Geometry: final body of the model. Coordinates: model frame, mm. Face numbers are marked on the shaded views. Round coordinates to 2 decimals unless told otherwise and drop trailing zeros. Order: outer loops, then holes, each group sorted by start corner. A loop starts at its lowest first (then second) coordinate and runs counter-clockwise, first axis right, second up. Notation, with made-up numbers: M 56.5,69 L 65.5,69 A21 cw 65.5,108 Z; hole C -24,-40 d5. An arc over 180 degrees is marked long. Put each result on its own line as item: value. Start each with the question number.
1) First-contact query: P1, Ø6.5, axis at x = 31.44, y = 9.74, coming from the -Z side; P2, Ø6.5, axis at x = 31.44, y = 9.74, coming from the +Z side; P3, Ø6, axis at x = 27, z = 3.5, coming from the +Y side; P4, Ø12, axis at y = 14, z = -4, coming from the -X side. Flat tips, straight axial feed; report the tip coordinate or a pass-through.
2) Section C-C, the plane y = 6.5. Return loops of the section in (x, z), then the cut area to 3 significant figures.
3) Section A-A, the plane x = 0. Return loops of the section in (y, z).
4) Material intervals for probe 1 along Z at (x, y) = (33, 18.75); probe 2 along Z at (x, y) = (0.5, 3.25); probe 3 along X at (y, z) = (7, 9), sorted ascending. Write a range as [from, to].
5) Section B-B, the plane z = -12.5. Return loops of the section in (x, y), then the cut area to 3 significant figures.
6) Draft query along Z for the marked faces 1, 2 and 3. Return one class per face: pulls with the +Z half, pulls with the -Z half, needs draft (parallel to the pull), parting line crosses it, or undercut.
from build123d import *

# Parameters (mm, degrees)
EXTRUDE_1_DEPTH       = 20
FILLET_1_R            = 2
FILLET_2_R            = 1
FILLET_3_R            = 5
HOLE_WIZARD_M51_D     = 4.2
HOLE_WIZARD_M51_DEPTH = 38.5
HOLE_WIZARD_M51_TIP   = 1.2618073


with BuildPart() as part:
    # Эскиз1 → Бобышка-Вытянуть1 (new body)
    with BuildSketch(Plane(origin=(0, 0, 0), x_dir=(1, 0, 0), z_dir=(0, 1, 0))):
        with BuildLine():
            Line((43.5, -1.5), (23.452078799, -1.5))
            ThreePointArc((23.452078799, -1.5), (-23.5, 0), (23.452078799, 1.5))
            Line((23.452078799, 1.5), (43.5, 1.5))
            Line((43.5, 1.5), (43.5, 0.5))
            Line((43.5, 0.5), (22.494443758, 0.5))
            ThreePointArc((22.494443758, 0.5), (-22.5, 0), (22.494443758, -0.5))
            Line((22.494443758, -0.5), (43.5, -0.5))
            Line((43.5, -0.5), (43.5, -1.5))
        make_face()
    extrude(amount=EXTRUDE_1_DEPTH)

    # Скругление1
    fillet_1_edges = [part.edges().sort_by_distance(p)[0] for p in [
        (22.494443758, 10, -0.5),
        (22.494443758, 10, 0.5),
    ]]
    fillet(fillet_1_edges, radius=FILLET_1_R)

    # Скругление2
    fillet_2_edges = [part.edges().sort_by_distance(p)[0] for p in [
        (23.452078799, 10, 1.5),
        (23.452078799, 10, -1.5),
    ]]
    fillet(fillet_2_edges, radius=FILLET_2_R)

    # Скругление3
    fillet_3_edges = [part.edges().sort_by_distance(p)[0] for p in [
        (43.5, 0, -1),
        (43.5, 20, 1),
        (43.5, 20, -1),
        (43.5, 0, 1),
    ]]
    fillet(fillet_3_edges, radius=FILLET_3_R)

    # Отверстие обработанное метчиком M51
    with Locations(Plane(origin=(0, 0, -1.5), x_dir=(-1, 0, 0), z_dir=(0, 0, -1))):
        with Locations((-31.436057607, 9.737709053)):
            Hole(HOLE_WIZARD_M51_D / 2, depth=HOLE_WIZARD_M51_DEPTH)
            with Locations((0, 0, -(HOLE_WIZARD_M51_DEPTH + HOLE_WIZARD_M51_TIP / 2))):  # 118° drill point
                Cone(0, HOLE_WIZARD_M51_D / 2, HOLE_WIZARD_M51_TIP, mode=Mode.SUBTRACT)


solid = part.part
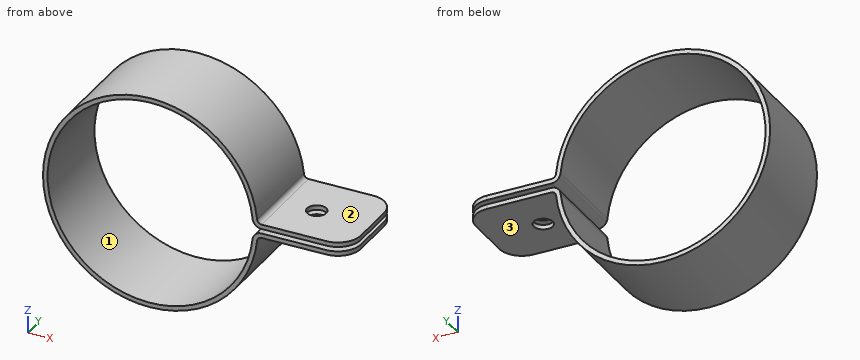
Result sheet:
1. P1: stops at z = -1.5
1. P2: stops at z = 1.5
1. P3: stops at y = 20
1. P4: stops at x = -23.5
2. outline: M 22.38,-2.3 A22.5 cw long 22.38,2.3 A2 ccw 24.37,0.5 L 43.5,0.5 L 43.5,1.5 L 24.37,1.5 A1 cw 23.38,2.4 A23.5 ccw long 23.38,-2.4 A1 cw 24.37,-1.5 L 43.5,-1.5 L 43.5,-0.5 L 24.37,-0.5 A2 ccw Z
2. area: 182 mm2
3. outline: M 0,-23.5 L 20,-23.5 L 20,-22.5 L 0,-22.5 Z; M 0,22.5 L 20,22.5 L 20,23.5 L 0,23.5 Z
4. probe 1: z = [-1.5, -0.5], [0.5, 1.5]
4. probe 2: z = [-23.49, -22.49], [22.49, 23.49]
4. probe 3: x = [-21.71, -20.62], [20.62, 21.71]
5. outline: M -19.9,0 L -18.71,0 L -18.71,20 L -19.9,20 Z; M 18.71,0 L 19.9,0 L 19.9,20 L 18.71,20 Z
5. area: 47.7 mm2
6. face 1: undercut
6. face 2: pulls with the +Z half
6. face 3: pulls with the -Z half
